```python
from build123d import *

# Parameters (mm, degrees)
F1_DEPTH = 25
F3_DEPTH = 5


with BuildPart() as f1:
    # F0 (on Front) → F1 (new body)
    with BuildSketch(Plane.XZ):
        with BuildLine():
            ThreePointArc((-43.08422, 24.874686), (-40.825433, 22.078816), (-41.025798, 18.490103))
            ThreePointArc((-41.025798, 18.490103), (0, -45), (41.025798, 18.490103))
            ThreePointArc((41.025798, 18.490103), (40.825433, 22.078816), (43.08422, 24.874686))
            ThreePointArc((43.08422, 24.874686), (45.472579, 28.154125), (44.642642, 32.125294))
            ThreePointArc((44.642642, 32.125294), (0, 55), (-44.642642, 32.125294))
            ThreePointArc((-44.642642, 32.125294), (-45.472579, 28.154125), (-43.08422, 24.874686))
        make_face()
        with BuildLine():
            ThreePointArc((-4.47822, -5.472253), (-2.785824, -4.868033), (-0.98911, -4.90119))
            ThreePointArc((-0.98911, -4.90119), (0, -5), (0.98911, -4.90119))
            ThreePointArc((0.98911, -4.90119), (2.785824, -4.868033), (4.47822, -5.472253))
            Line((4.47822, -5.472253), (28.356798, -19.258556))
            ThreePointArc((28.356798, -19.258556), (30.797764, -22.822617), (29.550627, -26.958495))
            ThreePointArc((29.550627, -26.958495), (0, -40), (-29.550627, -26.958495))
            ThreePointArc((-29.550627, -26.958495), (-30.797764, -22.822617), (-28.356798, -19.258556))
            Line((-28.356798, -19.258556), (-4.47822, -5.472253))
        make_face(mode=Mode.SUBTRACT)
        with BuildLine():
            ThreePointArc((-38.122055, -12.112346), (-34.641016, 20), (-8.571429, 39.070841))
            ThreePointArc((-8.571429, 39.070841), (-4.366084, 38.082954), (-2.5, 34.186986))
            Line((-2.5, 34.186986), (-2.5, 6.614378))
            ThreePointArc((-2.5, 6.614378), (-2.822928, 4.846611), (-3.75, 3.307189))
            ThreePointArc((-3.75, 3.307189), (-4.330127, 2.5), (-4.73911, 1.594001))
            ThreePointArc((-4.73911, 1.594001), (-5.608753, 0.021422), (-6.97822, -1.142126))
            Line((-6.97822, -1.142126), (-30.856798, -14.928429))
            ThreePointArc((-30.856798, -14.928429), (-35.163848, -15.260337), (-38.122055, -12.112346))
        make_face(mode=Mode.SUBTRACT)
        with BuildLine():
            ThreePointArc((3.75, 3.307189), (2.822928, 4.846611), (2.5, 6.614378))
            Line((2.5, 6.614378), (2.5, 34.186986))
            ThreePointArc((2.5, 34.186986), (4.366084, 38.082954), (8.571429, 39.070841))
            ThreePointArc((8.571429, 39.070841), (34.641016, 20), (38.122055, -12.112346))
            ThreePointArc((38.122055, -12.112346), (35.163848, -15.260337), (30.856798, -14.928429))
            Line((30.856798, -14.928429), (6.97822, -1.142126))
            ThreePointArc((6.97822, -1.142126), (5.608753, 0.021422), (4.73911, 1.594001))
            ThreePointArc((4.73911, 1.594001), (4.330127, 2.5), (3.75, 3.307189))
        make_face(mode=Mode.SUBTRACT)
    extrude(amount=F1_DEPTH)

    # F2 (on face) → F3 (cut)
    with BuildSketch(Plane.XZ.offset(25)):
        with BuildLine():
            ThreePointArc((-41.025798, 18.490103), (0, 45), (41.025798, 18.490103))
            ThreePointArc((41.025798, 18.490103), (40.825433, 22.078816), (43.08422, 24.874686))
            ThreePointArc((43.08422, 24.874686), (45.472579, 28.154125), (44.642642, 32.125294))
            ThreePointArc((44.642642, 32.125294), (0, 55), (-44.642642, 32.125294))
            ThreePointArc((-44.642642, 32.125294), (-45.472579, 28.154125), (-43.08422, 24.874686))
            ThreePointArc((-43.08422, 24.874686), (-40.825433, 22.078816), (-41.025798, 18.490103))
        make_face()
    extrude(amount=-F3_DEPTH, mode=Mode.SUBTRACT)


solid = f1.part
```
Model file for the job. Use its own axes, mm. A direction names the side the tool comes from. Coordinates: 2 decimals unless noted, no trailing zeros. Order: outer loops, then holes, each group sorted by start corner. A loop starts at its lowest first (then second) coordinate and runs counter-clockwise, first axis right, second up. Notation, with made-up numbers: (25, 7) -> (83, 7) arc R15 ccw to (83, 27) -> close; hole circle Ø7 at (54, -27.75). An arc over 180 degrees is marked (long way). Return JSON: item names as keys, results as strings.
Item 1: Slice it at B-B (x = -34). Write the cut outline in (y, z), then the cut area to 3 significant figures.
Model answer:
{"outline": "(-25, -29.48) -> (0, -29.48) -> (0, -15.56) -> (-25, -15.56) -> close; (-25, 21.07) -> (0, 21.07) -> (0, 43.23) -> (-20, 43.23) -> (-20, 29.48) -> (-25, 29.48) -> close", "area": "833 mm²"}
Item 2: Slice it at A-A (z = 5). Write the cut outline in (x, y), then the cut area to 3 significant figures.
Model answer:
{"outline": "(-44.72, -25) -> (-39.69, -25) -> (-39.69, 0) -> (-44.72, 0) -> close; (-2.77, -25) -> (2.77, -25) -> (2.77, 0) -> (-2.77, 0) -> close; (39.69, -25) -> (44.72, -25) -> (44.72, 0) -> (39.69, 0) -> close", "area": "390 mm²"}
Item 3: 3-axis set-ups, long thin cutter, end or side, ignore diameter. For faces 1 (the face through (2.761, -12.325, -4.864)), 2 (the face through (0, -25, 4)), 3 (the face through (-4, -20, 46)): which of +Z, -Z, +X, -X, +Y, -Y reach the whole face in a straight line?
Model answer:
{"face 1": "+Y, -Y", "face 2": "+Z, -Z, +X, -X, -Y", "face 3": "+Z, -Y"}
Item 4: Wall check: line 1 along Z through (x, y) = (22, -8.5); line 2 along X through (y, z) = (-20.5, -12.5); line 3 along Z through (x, y) = (29.5, -23). Give the ranges that are in metal, low to high. Write a range as from..to.
Model answer:
{"line 1": "z = -39.26..-33.41, -15.59..-9.81, 33.41..50.41", "line 2": "x = -43.23..-37.98, -26.65..-16.65, 16.65..26.65, 37.98..43.23", "line 3": "z = -33.98..-27.01, -20.16..-14.15, 27.01..33.98"}
Item 5: Pin check, flat tips, straight feed: P1, Ø1, axis at x = -9, y = -14.5, coming from the +Z side; P2, Ø10, axis at y = -9.5, z = -18.5, coming from the -X side; P3, Ø1.5, axis at x = -2.5, y = -3, coming from the +Z side. Stop position of each tip, or through.
Model answer:
{"P1": "stops at z = 54.34", "P2": "stops at x = -42.93", "P3": "stops at z = 54.97"}
Item 6: Mould opens along Z. For faces 4 (the face through (30.788, -12.325, -22.761)), 5 (the face through (-1, 0, 17)), 6 (the face through (-2.811, -12.325, -4.872)) say: pulls with the +Z half, pulls with the -Z half, needs draft (parallel to the pull), parting line crosses it, or undercut.
Model answer:
{"face 4": "undercut", "face 5": "needs draft", "face 6": "undercut"}
Item 7: Slice it at C-C (y = -1.25). Count the separate pieces of the cut face and the enclosed holes in it, then the cut area to 3 significant figures.
Model answer:
{"separate pieces": "1", "enclosed holes": "3", "area": "3,040 mm²"}
Item 8: Slice it at D-D (x = -16.5). Write the cut outline in (y, z), then the cut area to 3 significant figures.
Model answer:
{"outline": "(-25, -41.87) -> (0, -41.87) -> (0, -36.44) -> (-25, -36.44) -> close; (-25, -12.41) -> (0, -12.41) -> (0, -6.64) -> (-25, -6.64) -> close; (-25, 36.44) -> (0, 36.44) -> (0, 52.47) -> (-20, 52.47) -> (-20, 41.87) -> (-25, 41.87) -> close", "area": "628 mm²"}
